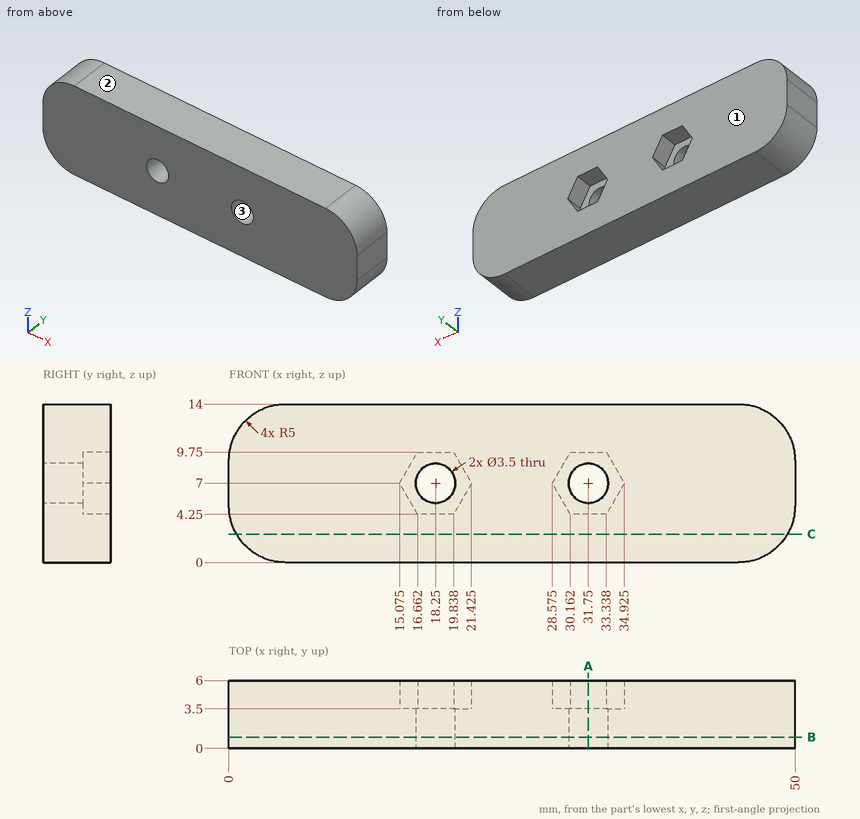
Check sheet for the drawn part. Datum: minimum x, y, z corner. Units: mm. Round coordinates to 2 decimals unless told otherwise and drop trailing zeros. Loops run counter-clockwise (first coordinate to the right, second up) from the corner with the lowest first, then second, coordinate; pieces in that order, holes last.
Item 1: Cross-section at A-A on x = 31.75. Record the boundary of the cut face in (y, z).
Item 2: Cross-section at C-C on z = 2.5. Record the boundary of the cut face in (x, y).
Item 3: Cross-section at B-B on y = 1. Record the boundary of the cut face in (x, z), then the cut area to 3 significant figures.
Item 4: Thickness scan on line 1 (X direction, y = 1.2, z = 7); line 2 (X direction, y = 2.55, z = 6.25); line 3 (Z direction, x = 18.25, y = 1.1). Record the ranges inside material, lowest first.
Item 5: Mould release check, pull along Z, two halves, no side actions. Record for the marked faces 1, 2 and 3: pulls with the +Z half, pulls with the -Z half, needs draft (parallel to the pull), parting line crosses it, or undercut.
Item 6: Gauge pin test, flat ends, axial feed: pin 1 (3 mm diameter, centred on y = 4.5, z = 11, fed in from -X) (1 decimal); pin 2 (1 mm diameter, centred on y = 1.5, z = 12.5, fed in from -X). Record the tip position at first contact, or that the pin passes through.
Answer sheet:
1. outline: (0, 0) - (6, 0) - (6, 4.25) - (3.5, 4.25) - (3.5, 5.25) - (0, 5.25) - close; (0, 8.75) - (3.5, 8.75) - (3.5, 9.75) - (6, 9.75) - (6, 14) - (0, 14) - close
2. outline: (0.67, 0) - (49.33, 0) - (49.33, 6) - (0.67, 6) - close
3. outline: (0, 5) arc R5 ccw to (5, 0) - (45, 0) arc R5 ccw to (50, 5) - (50, 9) arc R5 ccw to (45, 14) - (5, 14) arc R5 ccw to (0, 9) - close; hole circle Ø3.5 at (18.25, 7); hole circle Ø3.5 at (31.75, 7)
3. area: 659 mm2
4. line 1: x = 0 to 16.5, 20 to 30, 33.5 to 50
4. line 2: x = 0 to 16.67, 19.83 to 30.17, 33.33 to 50
4. line 3: z = 0 to 5.25, 8.75 to 14
5. face 1: needs draft
5. face 2: pulls with the +Z half
5. face 3: undercut
6. pin 1: stops at x = 0
6. pin 2: stops at x = 1
